```python
from build123d import *

# Parameters (mm, degrees)
SKETCH1_R           = 1.896742857
SKETCH1_R_2         = 1.45833049
SKETCH1_R_3         = 1.497428571
SKETCH1_R_4         = 2.695371429
BOSS_EXTRUDE1_DEPTH = 9.3865


with BuildPart() as part:
    # Sketch1 → Boss-Extrude1 (new, symmetric)
    with BuildSketch(Plane.XY):
        Polygon((-2.495714286, 15.780977349), (-11.230714286, 15.780977349), (-11.230714286, -20.77240592), (11.230714286, -20.77240592), (11.230714286, 15.780977349), (2.495714286, 15.780977349), (2.495714286, 20.77240592), (-2.495714286, 20.77240592), align=None)
        with Locations(Location((0, -6.680451222, 0), (0, 0, 180))):
            Circle(SKETCH1_R, mode=Mode.SUBTRACT)
        with Locations(Location((8.735, -15.964508365, 0), (0, 0, 180))):
            Circle(SKETCH1_R_2, mode=Mode.SUBTRACT)
        with Locations(Location((-8.735, -15.964508365, 0), (0, 0, 180))):
            Circle(SKETCH1_R_3, mode=Mode.SUBTRACT)
        with Locations(Location((0, 4.600177349, 0), (0, 0, 180))):
            Circle(SKETCH1_R_4, mode=Mode.SUBTRACT)
    extrude(amount=BOSS_EXTRUDE1_DEPTH, both=True)


solid = part.part
```
Can you work these out from the model? Positions are in its coordinate system, mm. A direction names the side the tool comes from. Coordinates: 2 decimals unless noted, no trailing zeros. Order: outer loops, then holes, each group sorted by start corner. A loop starts at its lowest first (then second) coordinate and runs counter-clockwise, first axis right, second up.
1. If we section it at C-C (x = -8.5): Please give me the cut outline in (y, z).
2. If we section it at A-A (x = 0): Please give me the cut outline in (y, z), then the cut area to 3 significant figures.
3. Thinking about a two-plate mould opening in Y: for faces 4 (the face through (-2.496, 18, 0)), 5 (the face through (7, 15.781, 0)), 6 (the face through (8.06, -14.67, -0.13)), 7 (the face through (0.25, -8.56, -0.13)), which applies, +Y half, -Y half, draft (parallel to the pull), parting line (faces both ways), or undercut?
4. I need wall thicknesses on line 1 (Y direction, x = 0, z = 5); line 2 (Y direction, x = -1, z = -3.75); line 3 (Y direction, x = -6, z = 7.5). Which ranges of each line are inside material? Lowest first, please.
5. I'm going to push flat-ended pins straight in: pin 1 (7 mm diameter, centred on x = 7, z = 2, fed in from +Y); pin 2 (2.5 mm diameter, centred on y = 18.5, z = -4.5, fed in from -X); pin 3 (2.5 mm diameter, centred on y = 19.5, z = 0, fed in from +X). Where does each tip first touch, or does it pass through?
6. If we section it at B-B (y = -15.5): Please give me the cut outline in (x, z), then the cut area to 3 significant figures.
7. If we section it at D-D (z = -4.5): Please give me the cut outline in (x, y) (1 decimal).
8. For faces 1 (the face through (-7, 15.781, 0)), 2 (the face through (11.231, -3, 0)), 3 (the face through (2.496, 18, 0)), which set-ups out of +Z, -Z, +X, -X, +Y, -Y let a thin tool reach every point of the face, with its end or its side?
Entries:
1. outline: (-20.77, -9.39) - (-17.44, -9.39) - (-17.44, 9.39) - (-20.77, 9.39) - close; (-14.49, -9.39) - (15.78, -9.39) - (15.78, 9.39) - (-14.49, 9.39) - close
2. outline: (-20.77, -9.39) - (-8.58, -9.39) - (-8.58, 9.39) - (-20.77, 9.39) - close; (-4.78, -9.39) - (1.9, -9.39) - (1.9, 9.39) - (-4.78, 9.39) - close; (7.3, -9.39) - (20.77, -9.39) - (20.77, 9.39) - (7.3, 9.39) - close
2. area: 608 mm2
3. face 4: draft
3. face 5: +Y half
3. face 6: undercut
3. face 7: undercut
4. line 1: y = -20.77 to -8.58, -4.78 to 1.9, 7.3 to 20.77
4. line 2: y = -20.77 to -8.29, -5.07 to 2.1, 7.1 to 20.77
4. line 3: y = -20.77 to 15.78
5. pin 1: stops at y = 15.78
5. pin 2: stops at x = -2.5
5. pin 3: stops at x = 2.5
6. outline: (-11.23, -9.39) - (-10.16, -9.39) - (-10.16, 9.39) - (-11.23, 9.39) - close; (-7.31, -9.39) - (7.35, -9.39) - (7.35, 9.39) - (-7.31, 9.39) - close; (10.12, -9.39) - (11.23, -9.39) - (11.23, 9.39) - (10.12, 9.39) - close
6. area: 316 mm2
7. outline: (-11.2, -20.8) - (11.2, -20.8) - (11.2, 15.8) - (2.5, 15.8) - (2.5, 20.8) - (-2.5, 20.8) - (-2.5, 15.8) - (-11.2, 15.8) - close; hole circle Ø3 at (-8.7, -16); hole circle Ø5.4 at (0, 4.6); hole circle Ø3.8 at (0, -6.7); hole circle Ø2.9 at (8.7, -16)
8. face 1: +Z, -Z, -X, +Y
8. face 2: +Z, -Z, +X, +Y, -Y
8. face 3: +Z, -Z, +X, +Y
